The model under review builds one solid part; all positions refer to its coordinate system, in mm. A direction names the side the tool comes from. Round coordinates to 2 decimals unless told otherwise and drop trailing zeros. Order: outer loops, then holes, each group sorted by start corner. A loop starts at its lowest first (then second) coordinate and runs counter-clockwise, first axis right, second up.
1) Consider section D-D (y = 19). Give the boundary of the cut face in (x, z).
2) Consider section B-B (x = 391.2). Give the boundary of the cut face in (y, z).
3) Consider section C-C (z = 11). Give the boundary of the cut face in (x, y), then the cut area to 3 significant figures.
4) Machinability: for faces 4 (the face through (375, 44, 23)), 5 (the face through (408, 44, -0.5)), 6 (the face through (389.202, 44.493, 10.912)), 7 (the face through (375, 44, -0.5)), which of the approach directions +Z, -Z, +X, -X, +Y, -Y give a long, thin tool a straight path to every point of the face, cutting with its end or side? Answer none if there is none.
5) Clearance check with flat-ended pins moving along their axes: P1, Ø0.6, axis at y = 43.5, z = -4.5, coming from the +X side; P2, Ø2, axis at x = 406.5, z = 25, coming from the +Y side; P3, Ø0.6, axis at x = 375, y = 44, coming from the -Z side. State where each tip first meets the part, or that it passes through.
6) Mouldability with a two-part tool opening along X and no side actions: class faces 1 (the face through (403.2, 44, -5)), 2 (the face through (395.97, 44.99, 9.5)), 3 (the face through (391, 9, 11)) as pulls with the +X half, pulls with the -X half, needs draft (parallel to the pull), parting line crosses it, or undercut.
7) Consider section A-A (z = 5). Give the boundary of the cut face in (x, y).
8) To check wall thickness, follow L1, parallel to Y at x = 408, z = 3.5; L2, parallel to Y at x = 392, z = 16. State the ranges of each line that lie inside material, in increasing order.
from build123d import *

# Parameters (mm, degrees)
CYLINDER007_R          = 2
CYLINDER007_DEPTH      = 36
CYLINDER007_ROLL_ANGLE = -90
CYLINDER004_R          = 5
CYLINDER004_DEPTH      = 31
CYLINDER004_ROLL_ANGLE = -90
CYLINDER002_R          = 10
CYLINDER002_DEPTH      = 11
CYLINDER002_ROLL_ANGLE = -90
CYLINDER003_R          = 5
CYLINDER003_DEPTH      = 19
CYLINDER003_ROLL_ANGLE = -90
CYLINDER001_R          = 5
CYLINDER001_DEPTH      = 31
CYLINDER001_ROLL_ANGLE = -90
BOX015_W               = 7.5
BOX015_H               = 3
BOX015_DEPTH           = 7.5
FILLET001_R            = 2
BOX017_W               = 7.5
BOX017_H               = 3
BOX017_DEPTH           = 7.5
FILLET002_R            = 2
BOX016_W               = 7.5
BOX016_H               = 3
BOX016_DEPTH           = 7.5
FILLET003_R            = 2
BOX014_W               = 7.5
BOX014_H               = 3
BOX014_DEPTH           = 7.5
FILLET_R               = 2
BOX012_W               = 38.5
BOX012_H               = 20
BOX012_DEPTH           = 38.5
CHAMFER_SIZE           = 2
CHAMFER001_1_SIZE      = 2
CHAMFER001_2_SIZE      = 1


with BuildPart() as eje_motor001:
    # Cylinder007 → Cylinder007 (new body)
    with BuildSketch(Plane.XY):
        Circle(CYLINDER007_R)
    extrude(amount=CYLINDER007_DEPTH)


with BuildPart() as eje_motor001_1:
    # Cylinder007 roll: moved
    add(eje_motor001.part.rotate(Axis((0, 0, 0), (1, 0, 0)), CYLINDER007_ROLL_ANGLE))


with BuildPart() as eje_motor001_2:
    # Cylinder007 placement: moved
    add(eje_motor001_1.part.moved(Location((379, 9, 11))))


with BuildPart() as cilindro015:
    # Cylinder004 → Cylinder004 (new body)
    with BuildSketch(Plane.XY):
        Circle(CYLINDER004_R)
    extrude(amount=CYLINDER004_DEPTH)


with BuildPart() as cilindro015_1:
    # Cylinder004 roll: moved
    add(cilindro015.part.rotate(Axis((0, 0, 0), (1, 0, 0)), CYLINDER004_ROLL_ANGLE))


with BuildPart() as cilindro015_2:
    # Cylinder004 placement: moved
    add(cilindro015_1.part.moved(Location((379, 55, 11))))


with BuildPart() as obj1:
    # Cylinder002 → Cylinder002 (new body)
    with BuildSketch(Plane.XY):
        Circle(CYLINDER002_R)
    extrude(amount=CYLINDER002_DEPTH)


with BuildPart() as obj1_1:
    # Cylinder002 roll: moved
    add(obj1.part.rotate(Axis((0, 0, 0), (1, 0, 0)), CYLINDER002_ROLL_ANGLE))


with BuildPart() as obj1_2:
    # Cylinder002 placement: moved
    add(obj1_1.part.moved(Location((379, 69, 11))))

    # Cut009: cut Cilindro015
    add(cilindro015_2.part, mode=Mode.SUBTRACT)


with BuildPart() as obj1_3:
    # Cut009 placement: moved
    add(obj1_2.part.moved(Location((0, -34, 0))))


with BuildPart() as dentro_motor:
    # Cylinder003 → Cylinder003 (new body)
    with BuildSketch(Plane.XY):
        Circle(CYLINDER003_R)
    extrude(amount=CYLINDER003_DEPTH)


with BuildPart() as dentro_motor_1:
    # Cylinder003 roll: moved
    add(dentro_motor.part.rotate(Axis((0, 0, 0), (1, 0, 0)), CYLINDER003_ROLL_ANGLE))


with BuildPart() as dentro_motor_2:
    # Cylinder003 placement: moved
    add(dentro_motor_1.part.moved(Location((379, 25, 11))))


with BuildPart() as cilindro012:
    # Cylinder001 → Cylinder001 (new body)
    with BuildSketch(Plane.XY):
        Circle(CYLINDER001_R)
    extrude(amount=CYLINDER001_DEPTH)


with BuildPart() as cilindro012_1:
    # Cylinder001 roll: moved
    add(cilindro012.part.rotate(Axis((0, 0, 0), (1, 0, 0)), CYLINDER001_ROLL_ANGLE))


with BuildPart() as cilindro012_2:
    # Cylinder001 placement: moved
    add(cilindro012_1.part.moved(Location((379, 21, 11))))


with BuildPart() as fillet001:
    # Box015 → Box015 (new body)
    with BuildSketch(Plane(origin=(391, 43, -8), x_dir=(1, 0, 0), z_dir=(0, 0, 1))):
        with Locations((3.75, 1.5)):
            Rectangle(BOX015_W, BOX015_H)
    extrude(amount=BOX015_DEPTH)

    # Fillet001
    fillet001_edges = [fillet001.edges().sort_by_distance(p)[0] for p in [
        (391, 44.5, -0.5),
    ]]
    fillet(fillet001_edges, radius=FILLET001_R)


with BuildPart() as fillet002:
    # Box017 → Box017 (new body)
    with BuildSketch(Plane(origin=(360, 43, -8), x_dir=(1, 0, 0), z_dir=(0, 0, 1))):
        with Locations((3.75, 1.5)):
            Rectangle(BOX017_W, BOX017_H)
    extrude(amount=BOX017_DEPTH)

    # Fillet002
    fillet002_edges = [fillet002.edges().sort_by_distance(p)[0] for p in [
        (367.5, 44.5, -0.5),
    ]]
    fillet(fillet002_edges, radius=FILLET002_R)


with BuildPart() as fillet003:
    # Box016 → Box016 (new body)
    with BuildSketch(Plane(origin=(360, 43, 23), x_dir=(1, 0, 0), z_dir=(0, 0, 1))):
        with Locations((3.75, 1.5)):
            Rectangle(BOX016_W, BOX016_H)
    extrude(amount=BOX016_DEPTH)

    # Fillet003
    fillet003_edges = [fillet003.edges().sort_by_distance(p)[0] for p in [
        (367.5, 44.5, 23),
    ]]
    fillet(fillet003_edges, radius=FILLET003_R)


with BuildPart() as fillet_body:
    # Box014 → Box014 (new body)
    with BuildSketch(Plane(origin=(391, 43, 23), x_dir=(1, 0, 0), z_dir=(0, 0, 1))):
        with Locations((3.75, 1.5)):
            Rectangle(BOX014_W, BOX014_H)
    extrude(amount=BOX014_DEPTH)

    # Fillet
    fillet_edges = [fillet_body.edges().sort_by_distance(p)[0] for p in [
        (391, 44.5, 23),
    ]]
    fillet(fillet_edges, radius=FILLET_R)


with BuildPart() as obj2:
    # Box012 → Box012 (new body)
    with BuildSketch(Plane(origin=(360, 25, -8), x_dir=(1, 0, 0), z_dir=(0, 0, 1))):
        with Locations((19.25, 10)):
            Rectangle(BOX012_W, BOX012_H)
    extrude(amount=BOX012_DEPTH)

    # Chamfer
    chamfer_edges = [obj2.edges().sort_by_distance(p)[0] for p in [
        (398.5, 35, 30.5),
    ]]
    chamfer(chamfer_edges, length=CHAMFER_SIZE)

    # Chamfer001 1
    chamfer001_1_edges = [obj2.edges().sort_by_distance(p)[0] for p in [
        (360, 35, 30.5),
    ]]
    chamfer(chamfer001_1_edges, length=CHAMFER001_1_SIZE)

    # Chamfer001 2
    chamfer001_2_edges = [obj2.edges().sort_by_distance(p)[0] for p in [
        (398.5, 35, -8),
        (360, 35, -8),
    ]]
    chamfer(chamfer001_2_edges, length=CHAMFER001_2_SIZE)

    # Cut005: cut Fillet body
    add(fillet_body.part, mode=Mode.SUBTRACT)

    # Cut006: cut Fillet003
    add(fillet003.part, mode=Mode.SUBTRACT)

    # Cut007: cut Fillet002
    add(fillet002.part, mode=Mode.SUBTRACT)

    # Cut008: cut Fillet001
    add(fillet001.part, mode=Mode.SUBTRACT)

    # Cut010: cut Cilindro012
    add(cilindro012_2.part, mode=Mode.SUBTRACT)

    # Fusion007: union obj1, dentro motor
    add(obj1_3.part)
    add(dentro_motor_2.part)

    # Fusion006: union eje motor001
    add(eje_motor001_2.part)


with BuildPart() as obj2_1:
    # Fusion006 placement: moved
    add(obj2.part.moved(Location((12.2, 0, 0))))


solid = obj2_1.part
Answer below:
1. outline: circle Ø4 at (391.2, 11)
2. outline: (9, 9) - (25, 9) - (25, -8) - (45, -8) - (45, 1) - (46, 1) - (46, 6) - (44, 6) - (44, 9) - (45, 9) - (45, 13) - (44, 13) - (44, 16) - (46, 16) - (46, 21) - (45, 21) - (45, 30.5) - (25, 30.5) - (25, 13) - (9, 13) - close
3. outline: (372.2, 25) - (389.2, 25) - (389.2, 9) - (393.2, 9) - (393.2, 25) - (410.7, 25) - (410.7, 45) - (401.2, 45) - (401.2, 46) - (396.2, 46) - (396.2, 44) - (393.2, 44) - (393.2, 45) - (389.2, 45) - (389.2, 44) - (386.2, 44) - (386.2, 46) - (381.2, 46) - (381.2, 45) - (372.2, 45) - close
3. area: 838 mm2
4. face 4: +Z, -X, +Y
4. face 5: -Z, +X, +Y
4. face 6: +Y
4. face 7: -Z, -X, +Y
5. P1: stops at x = 403.2
5. P2: stops at y = 43
5. P3: stops at z = -0.5
6. face 1: pulls with the +X half
6. face 2: undercut
6. face 3: needs draft
7. outline: (372.2, 25) - (410.7, 25) - (410.7, 45) - (399.2, 45) - (399.2, 46) - (383.2, 46) - (383.2, 45) - (372.2, 45) - close
8. L1: y = 25 to 45
8. L2: y = 25 to 46
